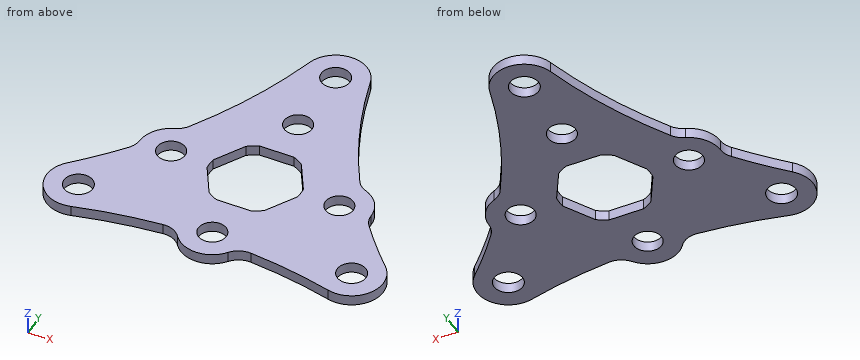
Autodesk Inventor part; units mm, degrees
ref_plane "YZ Plane" through (0, 0, 0) normal (1, 0, 0) x (0, 1, 0)
ref_plane "XZ Plane" through (0, 0, 0) normal (0, 1, 0) x (-1, 0, 0)
ref_plane "XY Plane" through (0, 0, 0) normal (0, 0, 1) x (1, 0, 0)
sketch "VersaHex Adapter Hole" plane through (0, 0, 0) normal (0, 0, 1) x (1, 0, 0)
  line L0 (-2.6931, -2.4859) -> (-0.0712, 2.0554)
  arc A0 (1.4952, 2.9597) -> (-0.0712, 2.0554) centre (4.1171, -3.3903) ccw
  line L1 (1.4952, 2.9597) -> (6.7391, 2.9597)
  arc A1 (8.3055, 2.0554) -> (6.7391, 2.9597) centre (4.1171, -3.3903) ccw
  line L2 (8.3055, 2.0554) -> (10.9274, -2.4859)
  arc A2 (10.9274, -4.2946) -> (10.9274, -2.4859) centre (4.1171, -3.3903) ccw
  line L3 (10.9274, -4.2946) -> (8.3055, -8.8359)
  arc A3 (6.7391, -9.7403) -> (8.3055, -8.8359) centre (4.1171, -3.3903) ccw
  line L4 (6.7391, -9.7403) -> (1.4952, -9.7403)
  arc A4 (-0.0712, -8.8359) -> (1.4952, -9.7403) centre (4.1171, -3.3903) ccw
  line L5 (-0.0712, -8.8359) -> (-2.6931, -4.2946)
  arc A5 (-2.6931, -2.4859) -> (-2.6931, -4.2946) centre (4.1171, -3.3903) ccw
  point P0 (3.8427, -3.1642)
  point P1 (0, 3.175)
  point P2 (0, -3.175)
  point P3 (0, 0)
sketch "Block2" plane through (0, 0, 0) normal (0, 0, 1) x (1, 0, 0)
  line L0 (30.4112, -18.6542) -> (33.0331, -14.1129)
  arc A0 (34.5995, -13.2085) -> (33.0331, -14.1129) centre (37.2214, -19.5585) ccw
  line L1 (34.5995, -13.2085) -> (39.8433, -13.2085)
  arc A1 (41.4097, -14.1129) -> (39.8433, -13.2085) centre (37.2214, -19.5585) ccw
  line L2 (41.4097, -14.1129) -> (44.0316, -18.6542)
  arc A2 (44.0316, -20.4629) -> (44.0316, -18.6542) centre (37.2214, -19.5585) ccw
  line L3 (44.0316, -20.4629) -> (41.4097, -25.0042)
  arc A3 (39.8433, -25.9085) -> (41.4097, -25.0042) centre (37.2214, -19.5585) ccw
  line L4 (39.8433, -25.9085) -> (34.5995, -25.9085)
  arc A4 (33.0331, -25.0042) -> (34.5995, -25.9085) centre (37.2214, -19.5585) ccw
  line L5 (33.0331, -25.0042) -> (30.4112, -20.4629)
  arc A5 (30.4112, -18.6542) -> (30.4112, -20.4629) centre (37.2214, -19.5585) ccw
  point P0 (37.2214, -19.5585)
sketch "Sketch1" plane through (0, 0, 0) normal (0, 0, 1) x (1, 0, 0)
  circle A0 centre (-20.6222, -11.9063) radius 2.1526
  circle A1 centre (20.6222, -11.9062) radius 2.1526
  circle A2 centre (0, 23.8125) radius 2.1526
  arc A3 (-24.0046, -8.5535) -> (-19.4099, -16.5119) centre (-20.6222, -11.9063) ccw
  arc A4 (19.4099, -16.5119) -> (24.0046, -8.5535) centre (20.6222, -11.9062) ccw
  arc A5 (4.5947, 25.0654) -> (-4.5947, 25.0654) centre (0, 23.8125) ccw
  arc A6 (-3.8147, -15.5513) -> (3.8147, -15.5513) centre (0, -12.7) ccw
  arc A7 (19.4099, -16.5119) -> (6.634, -14.2891) centre (0, -90.2489) ccw
  arc A8 (-6.634, -14.2891) -> (-19.4099, -16.5119) centre (0, -90.2489) ccw
  arc A9 (-3.8147, -15.5513) -> (-6.634, -14.2891) centre (-6.3578, -17.4521) ccw
  arc A10 (6.634, -14.2891) -> (3.8147, -15.5513) centre (6.3578, -17.4521) ccw
  circle A11 centre (0, -12.7) radius 2.0955
  circle A12 centre (0, 12.7) radius 2.0955
  circle A13 centre (-12.7, 0) radius 2.0955
  circle A14 centre (12.7, 0) radius 2.0955
  arc A15 (-14.4254, 4.439) -> (-17.4624, 0.0335) centre (-12.7, 0) ccw
  arc A16 (17.4624, 0.0335) -> (14.4254, 4.439) centre (12.7, 0) ccw
  arc A17 (-24.0046, -8.5535) -> (-18.1381, -1.9024) centre (-78.1579, 45.1245) ccw
  arc A18 (-12.8565, 5.7591) -> (-4.5947, 25.0654) centre (-78.1579, 45.1245) ccw
  arc A19 (4.5947, 25.0654) -> (12.8565, 5.7591) centre (78.1579, 45.1245) ccw
  arc A20 (18.1381, -1.9024) -> (24.0046, -8.5535) centre (78.1579, 45.1245) ccw
  arc A21 (-18.1381, -1.9024) -> (-17.4624, 0.0335) centre (-20.6373, 0.0558) ccw
  arc A22 (-14.4254, 4.439) -> (-12.8565, 5.7591) centre (-15.5756, 7.3983) ccw
  arc A23 (12.8565, 5.7591) -> (14.4254, 4.439) centre (15.5756, 7.3983) ccw
  arc A24 (17.4624, 0.0335) -> (18.1381, -1.9024) centre (20.6373, 0.0558) ccw
  line L0 (-6.8102, 0.9044) -> (-4.1883, 5.4456)
  arc A25 (-2.6219, 6.35) -> (-4.1883, 5.4456) centre (0, 0) ccw
  line L1 (-2.6219, 6.35) -> (2.6219, 6.35)
  arc A26 (4.1883, 5.4456) -> (2.6219, 6.35) centre (0, 0) ccw
  line L2 (4.1883, 5.4456) -> (6.8102, 0.9044)
  arc A27 (6.8102, -0.9044) -> (6.8102, 0.9044) centre (0, 0) ccw
  line L3 (6.8102, -0.9044) -> (4.1883, -5.4456)
  arc A28 (2.6219, -6.35) -> (4.1883, -5.4456) centre (0, 0) ccw
  line L4 (2.6219, -6.35) -> (-2.6219, -6.35)
  arc A29 (-4.1883, -5.4456) -> (-2.6219, -6.35) centre (0, 0) ccw
  line L5 (-4.1883, -5.4456) -> (-6.8102, -0.9044)
  arc A30 (-6.8102, 0.9044) -> (-6.8102, -0.9044) centre (0, 0) ccw
  dimension "d5" = 9.525
  dimension "d6" = 9.525
  dimension "d7" = 9.525
  dimension "d8" = 9.525
  dimension "d9" = 3.175
  dimension "d10" = 4.191
  dimension "d11" = 4.191
  dimension "d12" = 4.191
  dimension "d13" = 4.191
  dimension "d14" = 9.525
  dimension "d15" = 9.525
  dimension "d16" = 3.175
extrude "Extrusion1" add sketch "Sketch1" along normal blind 1.5875
equation "\"BendRadius\" = Thickness"
equation "\"BendReliefWidth\" = Thickness"
equation "\"BendReliefDepth\" = 0.5 * Thickness"
equation "\"CornerReliefSize\" = 4 * Thickness"
equation "\"MinimumRemnant\" = 2 * Thickness"
equation "\"TransitionRadius\" = BendRadius"
equation "\"JacobiRadiusSize\" = BendRadius"
equation "\"GapSize\" = Thickness"
properties part number "drop_center_hub" material "Acetal Resin, White"
Work out the finished part from the listing and answer in its coordinate system (mm). Coordinates: 2 decimals unless noted, no trailing zeros. Loops run counter-clockwise (first coordinate to the right, second up) from the corner with the lowest first, then second, coordinate; pieces in that order, holes last.
1) Section C-C (y = -12.7) is taken. Give the vertices of the cut face in (x, z), plus the area to 3 significant figures.
Results:
outline: (-25.32, 0) - (-22.62, 0) - (-22.62, 1.59) - (-25.32, 1.59) - close; (-18.62, 0) - (-2.1, 0) - (-2.1, 1.59) - (-18.62, 1.59) - close; (2.1, 0) - (18.62, 0) - (18.62, 1.59) - (2.1, 1.59) - close; (22.62, 0) - (25.32, 0) - (25.32, 1.59) - (22.62, 1.59) - close
area: 61.0 mm2
2) Section D-D (z = 0.25) is taken. Give the number of separate pieces and of enclosed holes in the cut face, plus the area to 3 significant figures.
Results:
separate pieces: 1
enclosed holes: 8
area: 986 mm2
3) A flat-ended cylindrical pin translates along its axis: pin 1 (2.5 mm diameter, centred on x = 0, y = 23.81, fed in from +Z). Find the tip coordinate at first contact, or state that the pin passes through.
Results:
pin 1: passes through
4) Section B-B (y = 12.7) is taken. Give the vertices of the cut face in (x, z).
Results:
outline: (-9.15, 0) - (-2.1, 0) - (-2.1, 1.59) - (-9.15, 1.59) - close; (2.1, 0) - (9.15, 0) - (9.15, 1.59) - (2.1, 1.59) - close
5) Section A-A (x = 0) is taken. Give the vertices of the cut face in (y, z).
Results:
outline: (-17.46, 0) - (-14.8, 0) - (-14.8, 1.59) - (-17.46, 1.59) - close; (-10.6, 0) - (-6.35, 0) - (-6.35, 1.59) - (-10.6, 1.59) - close; (6.35, 0) - (10.6, 0) - (10.6, 1.59) - (6.35, 1.59) - close; (14.8, 0) - (21.66, 0) - (21.66, 1.59) - (14.8, 1.59) - close; (25.97, 0) - (28.57, 0) - (28.57, 1.59) - (25.97, 1.59) - close
6) Consider probe 1 along X at (y, z) = (1, 1.5) (1 decimal); probe 2 along Y at (x, z) = (13.5, 0.25); probe 3 along X at (y, z) = (6, 0.7). Determine where each line is inside the solid, lowest interval first.
Results:
probe 1: x = -17.4 to -14.5, -10.9 to -6.8, 6.8 to 10.9, 14.5 to 17.4
probe 2: y = -15.2 to -1.94, 1.94 to 5
probe 3: x = -12.71 to -3.35, 3.35 to 12.71
